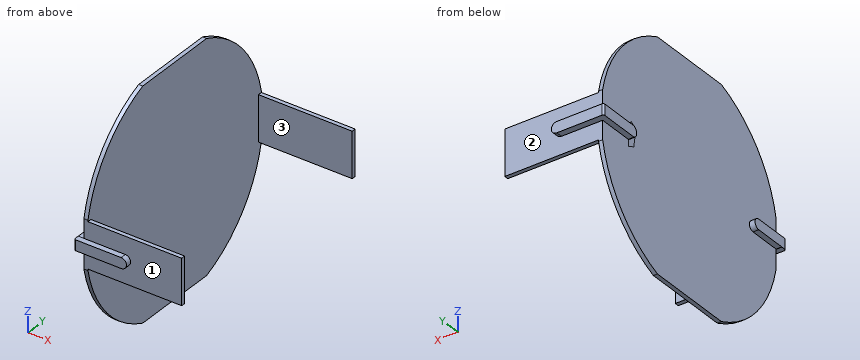
from build123d import *

# Parameters (mm, degrees)
ESBO_O1_R                   = 7.5
RESSALTO_EXTRUS_O1_DEPTH    = 6
ESBO_O2_W                   = 3
ESBO_O2_H                   = 0.472136223
CORTE_EXTRUS_O1_DEPTH       = 6
ESBO_O3_W                   = 2.966826726
ESBO_O3_H                   = 0.25
RESSALTO_EXTRUS_O2_DEPTH    = 5.75
ESBO_O4_W                   = 22.809874316
ESBO_O4_H                   = 14.203670942
CORTE_EXTRUS_O2_DEPTH       = 5.75
ESBO_O5_W                   = 7.250675024
ESBO_O5_H                   = 15.25065993
CORTE_EXTRUS_O3_DEPTH       = 10.75
RESSALTO_EXTRUS_O3_DEPTH    = 0.35
RESSALTO_EXTRUS_O4_DEPTH    = 0.35
CORTE_EXTRUS_O5_DEPTH       = 16
CORTE_EXTRUS_O5_DEPTH_BACK  = 6.35
CORTE_EXTRUS_O6_DEPTH       = 7.35
CORTE_EXTRUS_O6_DEPTH_BACK  = 13
FILETE1_R                   = 0.1
RESSALTO_EXTRUS_O5_DEPTH    = 0.4
CORTE_EXTRUS_O7_DEPTH       = 0.4
ESBO_O14_W                  = 0.349889087
ESBO_O14_H                  = 0.668418636
RESSALTO_EXTRUS_O6_DEPTH    = 2.4
FILETE2_R                   = 0.1
CORTE_EXTRUS_O9_DEPTH       = 0.35
CORTE_EXTRUS_O10_DEPTH      = 15
CORTE_EXTRUS_O10_DEPTH_BACK = 7.35


with BuildPart() as part:
    # Esboço1 → Ressalto-extrusão1 (new body)
    with BuildSketch(Plane(origin=(0, 0, 0), x_dir=(0, 0, -1), z_dir=(1, 0, 0))):
        Circle(ESBO_O1_R)
    extrude(amount=RESSALTO_EXTRUS_O1_DEPTH)

    # Esboço2 → Corte-extrusão1 (cut)
    with BuildSketch(Plane.ZY):
        with Locations((0, 7.587903583)):
            Rectangle(ESBO_O2_W, ESBO_O2_H)
        with Locations((0, -7.587903583)):
            Rectangle(ESBO_O2_W, ESBO_O2_H)
    extrude(amount=-CORTE_EXTRUS_O1_DEPTH, mode=Mode.SUBTRACT)

    # Esboço3 → Ressalto-extrusão2 (add)
    with BuildSketch(Plane.ZY):
        with Locations((0, 7.226835471)):
            Rectangle(ESBO_O3_W, ESBO_O3_H)
        with Locations((0, -7.226835471)):
            Rectangle(ESBO_O3_W, ESBO_O3_H)
    extrude(amount=-RESSALTO_EXTRUS_O2_DEPTH)

    # Esboço4 → Corte-extrusão2 (cut)
    with BuildSketch(Plane(origin=(6, 0, 0), x_dir=(0, 0, -1), z_dir=(1, 0, 0))):
        Rectangle(ESBO_O4_W, ESBO_O4_H)
    extrude(amount=-CORTE_EXTRUS_O2_DEPTH, mode=Mode.SUBTRACT)

    # Esboço5 → Corte-extrusão3 (cut)
    with BuildSketch(Plane(origin=(0.25, 0, 0), x_dir=(0, 0, -1), z_dir=(1, 0, 0))):
        with Locations((5.024783907, 0)):
            Rectangle(ESBO_O5_W, ESBO_O5_H)
        Polygon((-1.399446395, -7.625329965), (-1.399446395, 7.625329965), (-5.165706312, 7.393925443), (-6.710731139, 7.999984905), (-9.487585404, 6.78786598), (-11.382898632, -7.206597972), align=None)
    extrude(amount=CORTE_EXTRUS_O3_DEPTH, mode=Mode.SUBTRACT)

    # Esboço6 → Ressalto-extrusão3 (add)
    with BuildSketch(Plane.XZ.offset(7.351835471)):
        with BuildLine():
            Line((-2.543494754, 0.321961033), (2.543494754, 0.321961033))
            ThreePointArc((2.543494754, 0.321961033), (2.865455786, 0), (2.543494754, -0.321961033))
            Line((2.543494754, -0.321961033), (-2.543494754, -0.321961033))
            ThreePointArc((-2.543494754, -0.321961033), (-2.865455786, 0), (-2.543494754, 0.321961033))
        make_face()
    extrude(amount=RESSALTO_EXTRUS_O3_DEPTH)

    # Esboço8 → Ressalto-extrusão4 (add)
    with BuildSketch(Plane.ZY):
        with BuildLine():
            Line((-0.314307146, -9.305679126), (-0.314307146, -5.397991816))
            ThreePointArc((-0.314307146, -5.397991816), (0, -5.08368467), (0.314307146, -5.397991816))
            Line((0.314307146, -5.397991816), (0.314307146, -9.305679126))
            ThreePointArc((0.314307146, -9.305679126), (0, -9.619986272), (-0.314307146, -9.305679126))
        make_face()
    extrude(amount=RESSALTO_EXTRUS_O4_DEPTH)

    # Esboço9 → Corte-extrusão5 (cut, two sides: drawn at the far end of the back side and taken through both)
    with BuildSketch(Plane(origin=(0, 0, -0.321961033), x_dir=(-1, 0, 0), z_dir=(0, 0, -1)).offset(-CORTE_EXTRUS_O5_DEPTH_BACK)):
        Polygon((0.35, -7.701835471), (0.35, -4.813290401), (3.812040174, -6.789850405), (3.701673879, -8.068450161), (1.08322938, -8.435064851), align=None)
    extrude(amount=CORTE_EXTRUS_O5_DEPTH + CORTE_EXTRUS_O5_DEPTH_BACK, mode=Mode.SUBTRACT)

    # Esboço10 → Corte-extrusão6 (cut, two sides: drawn at the far end of the back side and taken through both)
    with BuildSketch(Plane(origin=(0, 0, -0.314307146), x_dir=(-1, 0, 0), z_dir=(0, 0, -1)).offset(-CORTE_EXTRUS_O6_DEPTH_BACK)):
        Polygon((-0.161358156, -7.701835471), (0.859566955, -7.701835471), (0.859566955, -10.409050105), (-1.096747377, -10.331004379), align=None)
    extrude(amount=CORTE_EXTRUS_O6_DEPTH + CORTE_EXTRUS_O6_DEPTH_BACK, mode=Mode.SUBTRACT)

    # Filete1
    filete1_edges = [part.edges().sort_by_distance(p)[0] for p in [
        (-0.35, -7.701835471, 0),
    ]]
    fillet(filete1_edges, radius=FILETE1_R)

    # Esboço11 → Ressalto-extrusão5 (add)
    with BuildSketch(Plane(origin=(0, 7.351835471, 0), x_dir=(1, 0, 0), z_dir=(0, 1, 0))):
        with BuildLine():
            Line((-2.525437349, 0.334209318), (2.525437349, 0.334209318))
            ThreePointArc((2.525437349, 0.334209318), (2.859646667, 0), (2.525437349, -0.334209318))
            Line((2.525437349, -0.334209318), (-2.525437349, -0.334209318))
            ThreePointArc((-2.525437349, -0.334209318), (-2.859646667, 0), (-2.525437349, 0.334209318))
        make_face()
    extrude(amount=RESSALTO_EXTRUS_O5_DEPTH)

    # Esboço13 → Corte-extrusão7 (cut)
    with BuildSketch(Plane(origin=(0, 7.751835471, 0), x_dir=(1, 0, 0), z_dir=(0, 1, 0))):
        Polygon((-0.349889087, -0.334209318), (-0.349889087, 0.540947425), (-0.764471769, 0.572838401), (-3.134268128, 0.417702141), (-3.23158757, -0.84745061), (0, -1.013091695), align=None)
    extrude(amount=-CORTE_EXTRUS_O7_DEPTH, mode=Mode.SUBTRACT)

    # Esboço14 → Ressalto-extrusão6 (add)
    with BuildSketch(Plane.XZ.offset(-7.351835471)):
        with Locations((-0.174944544, 0)):
            Rectangle(ESBO_O14_W, ESBO_O14_H)
    extrude(amount=RESSALTO_EXTRUS_O6_DEPTH)

    # Filete2
    filete2_edges = [part.edges().sort_by_distance(p)[0] for p in [
        (-0.349889087, 7.751835471, 0),
    ]]
    fillet(filete2_edges, radius=FILETE2_R)

    # Esboço15 → Corte-extrusão9 (cut)
    with BuildSketch(Plane.ZY.offset(0.349889087)):
        with BuildLine():
            Line((-0.334209318, 5.181370585), (-0.740677409, 5.181370585))
            Line((-0.740677409, 5.181370585), (-0.537443364, 4.71563988))
            Line((-0.537443364, 4.71563988), (0.580990807, 4.526830135))
            Line((0.580990807, 4.526830135), (0.857911766, 4.947135876))
            Line((0.857911766, 4.947135876), (0.334209318, 5.181370585))
            ThreePointArc((0.334209318, 5.181370585), (0, 4.947135876), (-0.334209318, 5.181370585))
        make_face()
    extrude(amount=-CORTE_EXTRUS_O9_DEPTH, mode=Mode.SUBTRACT)

    # Esboço19 → Corte-extrusão10 (cut, two sides: drawn at the far end of the back side and taken through both)
    with BuildSketch(Plane(origin=(0.25, 0, 0), x_dir=(0, 0, -1), z_dir=(1, 0, 0)).offset(-CORTE_EXTRUS_O10_DEPTH_BACK)):
        Polygon((-6.992682683, 8.188928042), (-12.721348099, -3.80184127), (-6.992682683, -8.188928042), align=None)
        Polygon((6.992682683, -8.188928042), (6.992682683, 8.188928042), (11.074646704, 2.193543386), align=None)
    extrude(amount=CORTE_EXTRUS_O10_DEPTH + CORTE_EXTRUS_O10_DEPTH_BACK, mode=Mode.SUBTRACT)


solid = part.part
Work out the finished part from the listing and answer in its coordinate system (mm). Face numbers are marked on the shaded views. Round coordinates to 2 decimals unless told otherwise and drop trailing zeros. Write each loop counter-clockwise with the first axis right and the second up, starting at its lowest first coordinate (ties: lowest second). Pieces come first, ordered by that corner, then holes. Notation, with made-up numbers: (8, 29.25) -> (48, 29.25) arc R23 cw to (48, 50.25) -> close; hole circle Ø4 at (65.5, 29.25). An arc over 180 degrees is marked (long way). Write each question's results on one line, items separated by ' | '.
Item 1: A cutting plane is placed at B-B, the plane x = 1.25. Determine the outline of the cut face in (y, z).
Result set:
outline: (-7.7, -0.32) -> (-7.35, -0.32) -> (-7.35, -1.4) -> (-7.1, -1.4) -> (-7.1, 1.4) -> (-7.35, 1.4) -> (-7.35, 0.32) -> (-7.7, 0.32) -> close; (7.1, -1.4) -> (7.35, -1.4) -> (7.35, -0.33) -> (7.75, -0.33) -> (7.75, 0.33) -> (7.35, 0.33) -> (7.35, 1.4) -> (7.1, 1.4) -> close
Item 2: Flat-ended cylindrical pins translate along their axes: P1, Ø2.5, axis at x = 4.5, z = 0.5, coming from the -Y side; P2, Ø1.3, axis at x = 1.5, y = 6.5, coming from the +Z side; P3, Ø1.5, axis at y = -0.5, z = -4.5, coming from the -X side. Find the tip coordinate at first contact, or state that the pin passes through.
Result set:
P1: y = -7.35 | P2: z = 1.4 | P3: x = 0
Item 3: Find the intervals of material crossed by line 1 along Y through (x, z) = (4.75, 0.5); line 2 along Y through (x, z) = (1, 0.25); line 3 along X through (y, z) = (-3.75, 5.75), in increasing order. Write a range as [from, to].
Result set:
line 1: [-7.35, -7.1], [7.1, 7.35] | line 2: [-7.7, -7.1], [7.1, 7.75] | line 3: [0, 0.25]
Item 4: A cutting plane is placed at A-A, the plane x = 5. Determine the outline of the cut face in (y, z).
Result set:
outline: (-7.35, -1.4) -> (-7.1, -1.4) -> (-7.1, 1.4) -> (-7.35, 1.4) -> close; (7.1, -1.4) -> (7.35, -1.4) -> (7.35, 1.4) -> (7.1, 1.4) -> close
Item 5: A cutting plane is placed at D-D, the plane y = 3. Determine the outline of the cut face in (x, z).
Result set:
outline: (0, -6.87) -> (0.25, -6.87) -> (0.25, 6.87) -> (0, 6.87) -> close
Item 6: The mould has two halves that part along Y. Classify the marked faces 1, 2 and 3: +Y half, -Y half, draft (parallel to the pull), parting line (faces both ways), or undercut.
Result set:
face 1: -Y half | face 2: +Y half | face 3: undercut
Item 7: A cutting plane is placed at C-C, the plane z = -2.5. Determine the outline of the cut face in (x, y).
Result set:
outline: (0, -7.07) -> (0.25, -7.07) -> (0.25, 7.07) -> (0, 7.07) -> close
